Here's how the part is built. I have some questions about the finished solid (model axes, mm). A direction names the side the tool comes from. Coordinates: 2 decimals unless noted, no trailing zeros. Loops run counter-clockwise (first coordinate to the right, second up) from the corner with the lowest first, then second, coordinate; pieces in that order, holes last. Notation, with made-up numbers: (2.5, 73.25) - (26.5, 73.25) arc R10 cw to (26.5, 82.25) - close; hole circle Ø1 at (-8.75, 7). An arc over 180 degrees is marked (long way). Use a Markdown table: item, result.
```python
from build123d import *

# Parameters (mm, degrees)
SKETCH1_W           = 76.14
SKETCH1_H           = 65.28
BOSS_EXTRUDE1_DEPTH = 80
SKETCH3_W           = 76.14
SKETCH3_H           = 65.28
SKETCH3_W_2         = 69.86
SKETCH3_H_2         = 59.89572892
BOSS_EXTRUDE2_DEPTH = 15
SKETCH4_W           = 70.14
SKETCH4_H           = 60.135791962
CUT_EXTRUDE1_DEPTH  = 75
SKETCH5_W           = 63.58
SKETCH5_H           = 54.51145784
BOSS_EXTRUDE3_DEPTH = 15


with BuildPart() as part:
    # Sketch1 → Boss-Extrude1 (new body)
    with BuildSketch(Plane(origin=(0, 0, 0), x_dir=(1, 0, 0), z_dir=(0, 1, 0))):
        Rectangle(SKETCH1_W, SKETCH1_H)
    extrude(amount=BOSS_EXTRUDE1_DEPTH)

    # Sketch3 → Boss-Extrude2 (add)
    with BuildSketch(Plane.XZ):
        Rectangle(SKETCH3_W, SKETCH3_H)
        Rectangle(SKETCH3_W_2, SKETCH3_H_2, mode=Mode.SUBTRACT)
    extrude(amount=BOSS_EXTRUDE2_DEPTH)

    # Sketch4 → Cut-Extrude1 (cut)
    with BuildSketch(Plane(origin=(0, 80, 0), x_dir=(1, 0, 0), z_dir=(0, 1, 0))):
        Rectangle(SKETCH4_W, SKETCH4_H)
    extrude(amount=-CUT_EXTRUDE1_DEPTH, mode=Mode.SUBTRACT)

    # Sketch5 → Boss-Extrude3 (add)
    with BuildSketch(Plane.XZ):
        Rectangle(SKETCH5_W, SKETCH5_H)
    extrude(amount=BOSS_EXTRUDE3_DEPTH)


solid = part.part
```
Q1. I want a section at B-B, the plane z = 23.5. Write out the boundary of the cut face in (x, y), then the cut area to 3 significant figures.
Check values:
| item | result |
|---|---|
| outline | (-38.07, -15) - (-34.93, -15) - (-34.93, 0) - (-31.79, 0) - (-31.79, -15) - (31.79, -15) - (31.79, 0) - (34.93, 0) - (34.93, -15) - (38.07, -15) - (38.07, 80) - (35.07, 80) - (35.07, 5) - (-35.07, 5) - (-35.07, 80) - (-38.07, 80) - close |
| area | 1,880 mm^2 |
Q2. Which directions (+Z, -Z, +X, -X, +Y, -Y) give clear straight access to the entire face, cutting with the end or side of a thin tool? Please do faces 5 (the face through (-34.93, -7, 0)), 6 (the face through (0, -15, 0)), 7 (the face through (0, 43, -30.068)).
Check values:
| item | result |
|---|---|
| face 5 | -Y |
| face 6 | +Z, -Z, +X, -X, -Y |
| face 7 | +Y |
Q3. Please list where these lines run through material, in increasing order: L1, parallel to Z at x = -25, y = 37.5; L2, parallel to Z at x = -14.5, y = -6.5; L3, parallel to X at y = 61.5, z = 18.5. Write a range as from..to.
Check values:
| item | result |
|---|---|
| L1 | -32.64..-30.07, 30.07..32.64 |
| L2 | -32.64..-29.95, -27.26..27.26, 29.95..32.64 |
| L3 | -38.07..-35.07, 35.07..38.07 |
Q4. I want a section at C-C, the plane x = 14.5. Write out the boundary of the cut face in (y, z), then the cut area to 3 significant figures.
Check values:
| item | result |
|---|---|
| outline | (-15, -32.64) - (80, -32.64) - (80, -30.07) - (5, -30.07) - (5, 30.07) - (80, 30.07) - (80, 32.64) - (-15, 32.64) - (-15, 29.95) - (0, 29.95) - (0, 27.26) - (-15, 27.26) - (-15, -27.26) - (0, -27.26) - (0, -29.95) - (-15, -29.95) - close |
| area | 1,610 mm^2 |
Q5. Will this pin go through, and if not, where does the flat tip stop? P1, Ø12, axis at x = 1.5, z = -5, coming from the +Y side.
Check values:
| item | result |
|---|---|
| P1 | y = 5 |
Q6. I want a section at A-A, the plane y = 55. Write out the boundary of the cut face in (x, z), then the cut area to 3 significant figures.
Check values:
| item | result |
|---|---|
| outline | (-38.07, -32.64) - (38.07, -32.64) - (38.07, 32.64) - (-38.07, 32.64) - close; hole (-35.07, -30.07) - (35.07, -30.07) - (35.07, 30.07) - (-35.07, 30.07) - close |
| area | 752 mm^2 |
Q7. If we mould it in two halves opening along Z, with no side actions, what happens to faces 1 (the face through (-1, 33, 32.64)), 2 (the face through (-1, 33, -32.64)), 3 (the face through (-38.07, 33, 0)), 4 (the face through (0, 5, 0))? For each: pulls with the +Z half, pulls with the -Z half, needs draft (parallel to the pull), parting line crosses it, or undercut.
Check values:
| item | result |
|---|---|
| face 1 | pulls with the +Z half |
| face 2 | pulls with the -Z half |
| face 3 | needs draft |
| face 4 | undercut |
